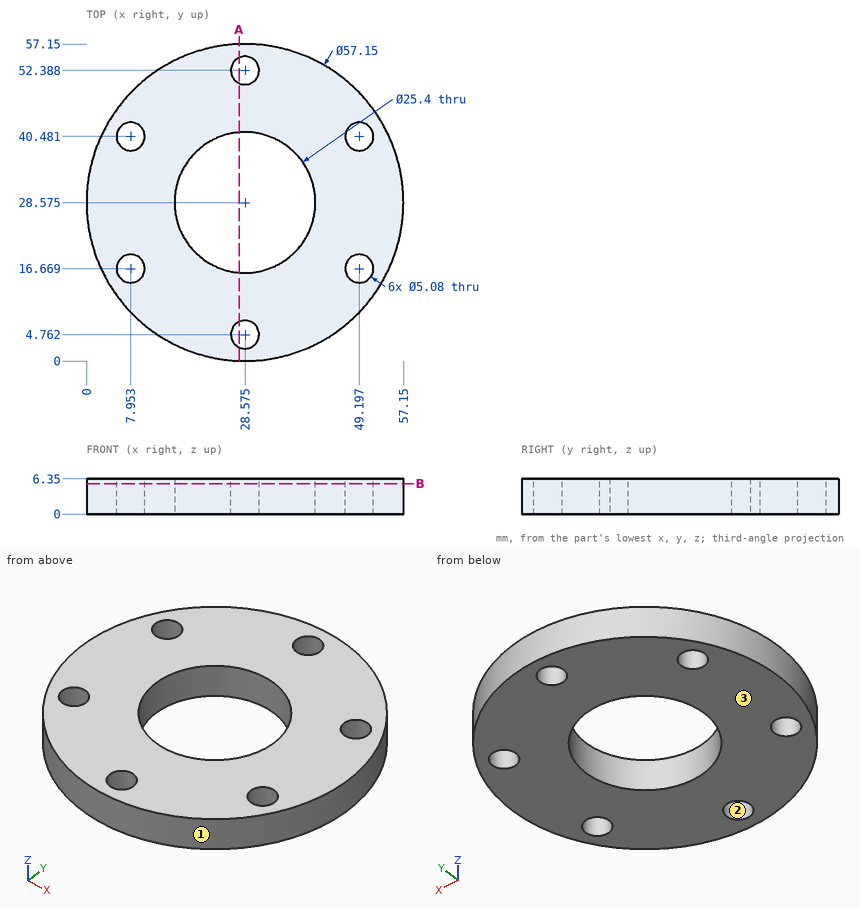
The drawing under review shows one solid part. Ordinate dimensions are in mm from its lowest x, y, z. Round coordinates to 2 decimals unless told otherwise and drop trailing zeros. Write each loop counter-clockwise with the first axis right and the second up, starting at its lowest first coordinate (ties: lowest second). Pieces come first, ordered by that corner, then holes. Notation, with made-up numbers: (4, 70.25) - (48, 70.25) arc R15 ccw to (48, 88.25) - close; hole circle Ø7 at (23, 26.25). An arc over 180 degrees is marked (long way). Use a Markdown table: item, result. Add a question column.
1. Mouldability with a two-part tool opening along X and no side actions: class the marked faces 1, 2 and 3 as +X half, -X half, draft (parallel to the pull), parting line (faces both ways), or undercut.
2. Wall thickness on probe 1 along X at (y, z) = (18.5, 1.75) (1 decimal); probe 2 along X at (y, z) = (18, 3.5) (1 decimal); probe 3 along X at (y, z) = (35, 3): over which ranges is each line inside the solid? List them lowest first.
3. Clearance check with flat-ended pins moving along their axes: pin 1 (6.5 mm diameter, centred on x = 49.2, y = 16.67, fed in from +Z); pin 2 (2 mm diameter, centred on y = 13, z = 2, fed in from +X); pin 3 (2 mm diameter, centred on y = 37.5, z = 4, fed in from +X). State where each tip first meets the part, or that it passes through.
4. We need section B-B (z = 5.5). Count the separate pieces of the cut face and the enclosed holes in it, then the cut area to 3 significant figures.
5. We need section A-A (x = 27.5). State the section outline as (y, z) points.
Output:
| question | item | result |
|---|---|---|
| 1 | face 1 | parting line |
| 1 | face 2 | undercut |
| 1 | face 3 | draft |
| 2 | probe 1 | x = 1.8 to 6.2, 9.7 to 20.8, 36.3 to 47.4, 51 to 55.3 |
| 2 | probe 2 | x = 2 to 5.8, 10.1 to 21.5, 35.6 to 47, 51.4 to 55.1 |
| 2 | probe 3 | x = 0.73 to 17.62, 39.53 to 56.42 |
| 3 | pin 1 | stops at z = 6.35 |
| 3 | pin 2 | stops at x = 53.15 |
| 3 | pin 3 | stops at x = 56.03 |
| 4 | separate pieces | 1 |
| 4 | enclosed holes | 7 |
| 4 | area | 1,940 mm2 |
| 5 | outline | (0.02, 0) - (2.46, 0) - (2.46, 6.35) - (0.02, 6.35) - close; (7.06, 0) - (15.92, 0) - (15.92, 6.35) - (7.06, 6.35) - close; (41.23, 0) - (50.09, 0) - (50.09, 6.35) - (41.23, 6.35) - close; (54.69, 0) - (57.13, 0) - (57.13, 6.35) - (54.69, 6.35) - close |
